from build123d import *

# Parameters (mm, degrees)
F1_DEPTH = 40
F2_W     = 20
F2_H     = 3
F3_DEPTH = 25
F4_R     = 3


with BuildPart() as f1:
    # F0 (on Top) → F1 (new body)
    with BuildSketch(Plane.XY):
        with BuildLine():
            Line((61.428977, 28.446451), (-58.221023, 28.446451))
            ThreePointArc((-58.221023, 28.446451), (-62.711151, 26.586579), (-64.571023, 22.096451))
            Line((-64.571023, 22.096451), (-64.571023, -18.203549))
            ThreePointArc((-64.571023, -18.203549), (-62.711151, -22.693677), (-58.221023, -24.553549))
            Line((-58.221023, -24.553549), (59.078977, -24.553549))
            ThreePointArc((59.078977, -24.553549), (63.569105, -22.693677), (65.428977, -18.203549))
            Line((65.428977, -18.203549), (65.428977, 24.446451))
            ThreePointArc((65.428977, 24.446451), (64.257404, 27.274878), (61.428977, 28.446451))
        make_face()
    extrude(amount=F1_DEPTH)

    # F2 (on face) → F3 (cut)
    with BuildSketch(Plane.XY.offset(40)):
        with Locations((-49.571023, 21.946451)):
            Rectangle(F2_W, F2_H)
        with Locations((-49.588825, 13.946471)):
            Rectangle(F2_W, F2_H)
        with Locations((-49.606627, 5.94649)):
            Rectangle(F2_W, F2_H)
        with Locations((-49.624429, -2.05349)):
            Rectangle(F2_W, F2_H)
        with Locations((-49.642231, -10.05347)):
            Rectangle(F2_W, F2_H)
        with Locations((-49.660033, -18.05345)):
            Rectangle(F2_W, F2_H)
        with Locations((-24.571023, 21.946451)):
            Rectangle(F2_W, F2_H)
        with Locations((-24.588825, 13.946471)):
            Rectangle(F2_W, F2_H)
        with Locations((-24.606627, 5.94649)):
            Rectangle(F2_W, F2_H)
        with Locations((-24.624429, -2.05349)):
            Rectangle(F2_W, F2_H)
        with Locations((-24.642231, -10.05347)):
            Rectangle(F2_W, F2_H)
        with Locations((-24.660033, -18.05345)):
            Rectangle(F2_W, F2_H)
        with Locations((0.428977, 21.946451)):
            Rectangle(F2_W, F2_H)
        with Locations((0.411175, 13.946471)):
            Rectangle(F2_W, F2_H)
        with Locations((0.393373, 5.94649)):
            Rectangle(F2_W, F2_H)
        with Locations((0.375571, -2.05349)):
            Rectangle(F2_W, F2_H)
        with Locations((0.357769, -10.05347)):
            Rectangle(F2_W, F2_H)
        with Locations((0.339967, -18.05345)):
            Rectangle(F2_W, F2_H)
        with Locations((25.428977, 21.946451)):
            Rectangle(F2_W, F2_H)
        with Locations((25.411175, 13.946471)):
            Rectangle(F2_W, F2_H)
        with Locations((25.393373, 5.94649)):
            Rectangle(F2_W, F2_H)
        with Locations((25.375571, -2.05349)):
            Rectangle(F2_W, F2_H)
        with Locations((25.357769, -10.05347)):
            Rectangle(F2_W, F2_H)
        with Locations((25.339967, -18.05345)):
            Rectangle(F2_W, F2_H)
        with Locations((50.428977, 21.946451)):
            Rectangle(F2_W, F2_H)
        with Locations((50.411175, 13.946471)):
            Rectangle(F2_W, F2_H)
        with Locations((50.393373, 5.94649)):
            Rectangle(F2_W, F2_H)
        with Locations((50.375571, -2.05349)):
            Rectangle(F2_W, F2_H)
        with Locations((50.357769, -10.05347)):
            Rectangle(F2_W, F2_H)
        with Locations((50.339967, -18.05345)):
            Rectangle(F2_W, F2_H)
    extrude(amount=-F3_DEPTH, mode=Mode.SUBTRACT)

    # F4
    f4_edges = [f1.edges().sort_by_distance(p)[0] for p in [
        (1.603977, 28.446451, 40),
    ]]
    fillet(f4_edges, radius=F4_R)


solid = f1.part
Verification items for the finished model (mm, model axes). Give positions to 0.01 mm unless a question says otherwise; leave off trailing zeros.
1) Sectioned sample at B-B, the plane z = 34. Count the separate pieces of the cut face and the enclosed holes in it, then the cut area to 3 significant figures.
2) Thickness scan on line 1 along X through (y, z) = (-17, 38); line 2 along X through (y, z) = (23, 38); line 3 along Z through (x, y) = (-48, 13.5). Record the ranges inside material, lowest first.
3) Draft check along Y on faces 1 (the flat face through (15.411, 14, 28)), 2 (the flat face through (2, 28.446, 18)). Enter one of: pulls with the +Y half, pulls with the -Y half, needs draft (parallel to the pull), parting line crosses it, or undercut.
4) Depth check by flat-ended pin: pin 1 Ø2.5 at (x, y) = (-20.5, 6) entering from +Z. Enter the tip coordinate at first touch or a pass-through.
Answers:
1. separate pieces: 1
1. enclosed holes: 30
1. area: 5,060 mm2
2. line 1: x = -64.4 to -59.66, -39.66 to -34.66, -14.66 to -9.66, 10.34 to 15.34, 35.34 to 40.34, 60.34 to 65.26
2. line 2: x = -64.33 to -59.57, -39.57 to -34.57, -14.57 to -9.57, 10.43 to 15.43, 35.43 to 40.43, 60.43 to 65.26
2. line 3: z = 0 to 15
3. face 1: undercut
3. face 2: pulls with the +Y half
4. pin 1: stops at z = 15
